Part model, mm, in its own coordinate system. A direction names the side the tool comes from. Coordinates: 2 decimals unless noted, no trailing zeros. Order: outer loops, then holes, each group sorted by start corner. A loop starts at its lowest first (then second) coordinate and runs counter-clockwise, first axis right, second up.
```python
from build123d import *

# Parameters (mm, degrees)
LED_1_OUTLINE_R     = 2.25
LED_1_DEPTH         = 3
SKETCH_1_W          = 100
SKETCH_1_H          = 9
CUT_EXTRUDE_1_DEPTH = 3


# Read off the part's stored shape, not the designer's step: 基体零件-LED板-1
with BuildPart() as part:
    # 基体零件-LED板-1 outline → 基体零件-LED板-1 (new body)
    with BuildSketch(Plane(origin=(0, 0, 0), x_dir=(1, 0, 0), z_dir=(0, 1, 0))):
        Polygon((-3, -140), (0, -140), (0, -110), (-3, -110), (-3, -100), (-115, -100), (-115, -110), (-118, -110), (-118, -140), (-115, -140), (-115, -150), (-6.001970153, -150), (-6.001970153, -144), (-3, -144), align=None)
        with Locations((-90.5, -130)):
            Circle(LED_1_OUTLINE_R, mode=Mode.SUBTRACT)
        with Locations((-81.5, -130)):
            Circle(LED_1_OUTLINE_R, mode=Mode.SUBTRACT)
        with Locations((-72.5, -130)):
            Circle(LED_1_OUTLINE_R, mode=Mode.SUBTRACT)
        with Locations((-63.5, -130)):
            Circle(LED_1_OUTLINE_R, mode=Mode.SUBTRACT)
        with Locations((-54.5, -130)):
            Circle(LED_1_OUTLINE_R, mode=Mode.SUBTRACT)
        with Locations((-45.5, -130)):
            Circle(LED_1_OUTLINE_R, mode=Mode.SUBTRACT)
        with Locations((-36.5, -130)):
            Circle(LED_1_OUTLINE_R, mode=Mode.SUBTRACT)
        with Locations((-27.5, -130)):
            Circle(LED_1_OUTLINE_R, mode=Mode.SUBTRACT)
    extrude(amount=LED_1_DEPTH)

    # 草图1 → 切除-拉伸1 (cut)
    with BuildSketch(Plane(origin=(0, 3, 0), x_dir=(1, 0, 0), z_dir=(0, 1, 0))):
        with Locations((-59, -130)):
            Rectangle(SKETCH_1_W, SKETCH_1_H)
    extrude(amount=-CUT_EXTRUDE_1_DEPTH, mode=Mode.SUBTRACT)


solid = part.part
```
(1) Tool access for faces 5 (the face through (-117, 1, 140)), 6 (the face through (-5, 1, 144)), 7 (the face through (-115, 1, 105)), 8 (the face through (-1, 1, 110)), 9 (the face through (-60, 2, 125.5)): list every direction of +Z, -Z, +X, -X, +Y, -Y with a clear straight run to the whole face (end or side of a thin tool).
(2) Pull direction Z, two halves, no side cores. Call faces 1 (the face through (-2, 1, 140)), 2 (the face through (-116, 1, 110)), 3 (the face through (-115, 1, 145)), 4 (the face through (-109, 2, 130)): +Z half, -Z half, draft (parallel to the pull), parting line (faces both ways), or undercut.
(3) Drop flat-ended pins along their axis: pin 1 (1.5 mm diameter, centred on y = 1, z = 146, fed in from +X); pin 2 (0.9 mm diameter, centred on y = 2, z = 143.5, fed in from -X); pin 3 (0.9 mm diameter, centred on x = -117, y = 1, fed in from +Z). Give the stop position or say it passes through.
(4) Slice it at B-B, the plane z = 133. Give the cut face in (x, y).
(5) Slice it at C-C, the plane y = 1.1. Give the cut face in (x, z), then the cut area to 3 significant figures.
(6) Probe line 1 (Z direction, x = -68.5, y = 0.65); line 2 (X direction, y = 0.35, z = 131); line 3 (X direction, y = 2.4, z = 145). List the from-to ranges inside material, lowest first.
(7) Slice it at D-D, the plane z = 142.5. Give the cut face in (x, y), then the cut area to 3 significant figures.
(8) Slice it at A-A, the plane x = -10.5. Give the cut face in (y, z), then the cut area to 3 significant figures.
Here are the results:
1. face 5: +Z, -X, +Y, -Y
1. face 6: +Z, +X, +Y, -Y
1. face 7: -Z, -X, +Y, -Y
1. face 8: -Z, +X, +Y, -Y
1. face 9: +Y, -Y
2. face 1: +Z half
2. face 2: -Z half
2. face 3: draft
2. face 4: undercut
3. pin 1: stops at x = -6
3. pin 2: stops at x = -115
3. pin 3: stops at z = 140
4. outline: (-118, 0) - (-109, 0) - (-109, 3) - (-118, 3) - close; (-9, 0) - (0, 0) - (0, 3) - (-9, 3) - close
5. outline: (-118, 110) - (-115, 110) - (-115, 100) - (-3, 100) - (-3, 110) - (0, 110) - (0, 140) - (-3, 140) - (-3, 144) - (-6, 144) - (-6, 150) - (-115, 150) - (-115, 140) - (-118, 140) - close; hole (-109, 125.5) - (-9, 125.5) - (-9, 134.5) - (-109, 134.5) - close
5. area: 4,860 mm2
6. line 1: z = 100 to 125.5, 134.5 to 150
6. line 2: x = -118 to -109, -9 to 0
6. line 3: x = -115 to -6
7. outline: (-115, 0) - (-3, 0) - (-3, 3) - (-115, 3) - close
7. area: 336 mm2
8. outline: (0, 100) - (3, 100) - (3, 125.5) - (0, 125.5) - close; (0, 134.5) - (3, 134.5) - (3, 150) - (0, 150) - close
8. area: 123 mm2
